Read the model definition and answer for the solid it produces. Units are mm, in the model's axes. Face numbers are marked on the shaded views. A direction names the side the tool comes from. Coordinates: 2 decimals unless noted, no trailing zeros. Loops run counter-clockwise (first coordinate to the right, second up) from the corner with the lowest first, then second, coordinate; pieces in that order, holes last. Notation, with made-up numbers: M 11.25,-39 L 36.25,-39 A17 ccw 36.25,-17 Z; hole C 48,-1.75 d5. An arc over 180 degrees is marked long. Use one line per item in the form item = value. Start each with the question number.
1. A tool of negligible diameter and unlimited length cuts with its end or side. For the marked faces 5, 6, 7 and 8, from which of +Z, -Z, +X, -X, +Y, -Y can it reach the whole face along a straight path? Write none if from no direction.
2. The part is cut by section B-B (z = 4.5). Give the vertices of the cut face in (x, y), plus the area to 3 significant figures.
3. Flat-ended cylindrical pins translate along their axes: pin 1 (3 mm diameter, centred on y = 20, z = 6, fed in from -X); pin 2 (1.5 mm diameter, centred on x = 25, z = -9.5, fed in from +Y); pin 3 (9 mm diameter, centred on y = 13, z = -6.5, fed in from +X); pin 4 (6 mm diameter, centred on x = 8, z = 2, fed in from -Y). Find the tip coordinate at first contact, or state that the pin passes through.
4. The part is cut by section D-D (y = 19.5). Give the vertices of the cut face in (x, z), plus the area to 3 significant figures.
5. The part is cut by section A-A (y = -12). Give the vertices of the cut face in (x, z), plus the area to 3 significant figures.
6. Find the intervals of material crossed by probe 1 along X at (y, z) = (-12, -10); probe 2 along Y at (x, z) = (36.75, 0); probe 3 along Y at (x, z) = (11, -2.5), in increasing order. Write a range as [from, to].
7. For a pull along Y with two mould halves and no side action, classify the marked faces 1, 2, 3 and 4 as released by +Y, released by -Y, zero draft, split by the parting line, or undercut.
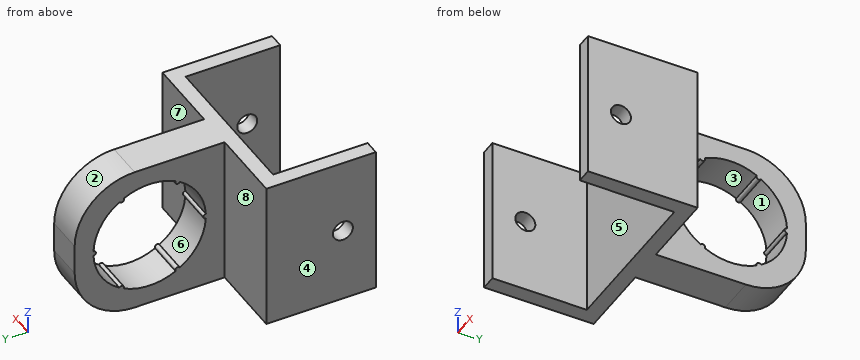
Autodesk Inventor part; units mm, degrees
ref_plane "YZ Plane" through (0, 0, 0) normal (1, 0, 0) x (0, 1, 0)
ref_plane "XZ Plane" through (0, 0, 0) normal (0, 1, 0) x (-1, 0, 0)
ref_plane "XY Plane" through (0, 0, 0) normal (0, 0, 1) x (1, 0, 0)
sketch "Sketch2" plane through (0, 0, 0) normal (0, 0, 1) x (1, 0, 0)
  line L0 (31.3357, -4.795) -> (6.3357, -4.795)
  line L1 (6.3357, -4.795) -> (6.3357, -1.5952)
  line L2 (31.3357, -1.5952) -> (6.3357, -1.5952)
  line L3 (31.3357, -4.795) -> (31.3357, -1.5952)
  line L4 (6.3357, -1.5952) -> (6.3357, -21.5944)
  line L5 (6.3357, -21.5944) -> (3.1357, -21.5944)
  line L6 (3.1357, -1.5952) -> (3.1357, -21.5944)
  line L7 (6.3357, -1.5952) -> (3.1357, -1.5952)
  line L8 (31.3357, -21.5944) -> (31.3357, -1.5952)
  line L9 (31.3357, -1.5952) -> (34.5357, -1.5952)
  line L10 (34.5357, -21.5944) -> (34.5357, -1.5952)
  line L11 (31.3357, -21.5944) -> (34.5357, -21.5944)
  line L12 (6.3357, -23.8087) -> (3.1357, -23.8087)
  line L13 (34.8357, -21.5944) -> (34.8357, -2.6826)
  line L14 (34.8357, -21.5944) -> (37.8357, -21.5944)
  line L15 (37.8357, -21.5944) -> (37.8357, 0.3174)
  line L16 (18.8357, -1.5952) -> (18.8357, -12.9026) construction
  line L17 (2.8357, -21.5944) -> (2.8357, -2.6826)
  line L18 (2.8357, -21.5944) -> (-0.1643, -21.5944)
  line L19 (-0.1643, -21.5944) -> (-0.1643, 0.3174)
  line L20 (2.8357, -2.6826) -> (34.8357, -2.6826)
  line L21 (-0.1643, 0.3174) -> (37.8357, 0.3174)
  line L22 (22.5857, 0.3174) -> (22.5857, 30.3174)
  line L23 (22.5857, 30.3174) -> (15.0857, 30.3174)
  line L24 (15.0857, 30.3174) -> (15.0857, 0.3174)
  line L25 (6.3357, -2.9826) -> (31.3357, -2.9826)
  point P0 (0, 0)
  dimension "d1" = 0.3
  dimension "d2" = 3
  dimension "d5" = 32
  dimension "d9" = 30
  dimension "d10" = 7.5
  dimension "d11" = 3.75
  dimension "d18" = 0.3
  dimension "d19" = 3
extrude "Extrusion1" add sketch "Sketch2" along normal mid plane 30 contours L20 L1 L2 L3 | L3 L9 L10 L20 | L20 L6 L7 L1 | L2 L7 L6 L20 L17 L18 L19 L21 L15 L14 L13 L10 L9 | L21 L24 L23 L22
sketch "Sketch3" plane through (37.8357, -21.5944, 15) normal (1, 0, 0) x (0, 0, -1)
  circle A0 centre (13.5169, 6.5933) radius 2
  line L0 (30, 21.9118) -> (30, 0)
  line L1 (0, 0) -> (0, 21.9118)
  line L2 (30, 0) -> (0, 0)
  line L3 (0, 21.9118) -> (30, 21.9118)
  line L4 (30, 0) -> (0, 0)
  line L5 (15, 0) -> (15, 21.9118) construction
  circle A1 centre (15, 6.5933) radius 2
  point P0 (15, 21.5944)
  dimension "d14" = 4
  dimension "d15" = 6.5933
extrude "Extrusion2" cut sketch "Sketch3" against normal blind 60 contours A0 A1 | A0 A1 picked at (14.6591, 6.7506) picked at (16.4859, 6.7542)
sketch "Sketch4" plane through (15.0857, 0.3174, 15) normal (-1, 0, 0) x (0, 0, 1)
  line L0 (-30, 0) -> (0, 0)
  line L1 (0, 30) -> (0, 0)
  line L2 (-30, 30) -> (0, 30)
  line L3 (-30, 0) -> (-30, 30)
  line L4 (-30, 0) -> (0, 0)
  line L5 (-15, 0) -> (-15, 30) construction
  line L6 (-30, 30) -> (0, 30)
  line L7 (0, 0) -> (0, 30)
  line L8 (0, 15) -> (-30, 15) construction
  circle A0 centre (-15, 15) radius 11.25
  arc A1 (-14.5001, 3.7611) -> (-15.4999, 3.7611) centre (-15, 3.75) ccw
  arc A2 (-5.0169, 9.8135) -> (-5.5168, 8.9476) centre (-5.2572, 9.375) ccw
  arc A3 (-5.5168, 21.0524) -> (-5.0169, 20.1865) centre (-5.2572, 20.625) ccw
  arc A4 (-15.4999, 26.2389) -> (-14.5001, 26.2389) centre (-15, 26.25) ccw
  arc A5 (-24.9831, 20.1865) -> (-24.4832, 21.0524) centre (-24.7428, 20.625) ccw
  arc A6 (-24.4832, 8.9476) -> (-24.9831, 9.8135) centre (-24.7428, 9.375) ccw
  point P0 (-15, -0.3174)
  point P1 (-24.9831, 9.8135)
  point P2 (-24.4832, 8.9476)
  point P3 (-5.5168, 8.9476)
  point P4 (-5.0169, 9.8135)
  point P5 (-5.0169, 20.1865)
  point P6 (-5.5168, 21.0524)
  point P7 (-14.5001, 26.2389)
  point P8 (-15.4999, 26.2389)
  point P9 (-24.4832, 21.0524)
  point P10 (-24.9831, 20.1865)
  dimension "d20" = 22.5
  dimension "d21" = 1
  dimension "d24" = 360
extrude "Extrusion3" cut sketch "Sketch4" against normal blind 10 contours A0 A2 A1 A6 A5 A4 A3
fillet "Fillet1" radius 12 2 edges at (18.8357, 30.3174, 15) (18.8357, 30.3174, -15)
properties part number "Eje_Carril"
Computed values:
q1.face_5 = +Z, -Z, -Y
q1.face_6 = +X, -X
q1.face_7 = +Z, -Z, +X, +Y
q1.face_8 = +Z, -Z, -X, +Y
q2.outline = M -0.16,-21.59 L 2.84,-21.59 L 2.84,-2.68 L 34.84,-2.68 L 34.84,-21.59 L 37.84,-21.59 L 37.84,0.32 L 22.59,0.32 L 22.59,5.01 L 15.09,5.01 L 15.09,0.32 L -0.16,0.32 Z; M 15.09,25.63 L 22.59,25.63 L 22.59,30.22 L 15.09,30.22 Z
q2.area = 297 mm²
q3.pin_1 = through
q3.pin_2 = 0.32
q3.pin_3 = 22.59
q3.pin_4 = -2.68
q4.outline = M 15.09,-14.94 L 22.59,-14.94 L 22.59,-10.44 L 15.09,-10.44 Z; M 15.09,10.44 L 22.59,10.44 L 22.59,14.94 L 15.09,14.94 Z
q4.area = 67.5 mm²
q5.outline = M -0.16,-15 L 2.84,-15 L 2.84,15 L -0.16,15 Z; M 34.84,-15 L 37.84,-15 L 37.84,15 L 34.84,15 Z
q5.area = 180 mm²
q6.probe_1 = [-0.16, 2.84], [34.84, 37.84]
q6.probe_2 = [-21.59, -17], [-13, 0.32]
q6.probe_3 = [-2.68, 0.32]
q7.face_1 = undercut
q7.face_2 = released by +Y
q7.face_3 = undercut
q7.face_4 = zero draft
